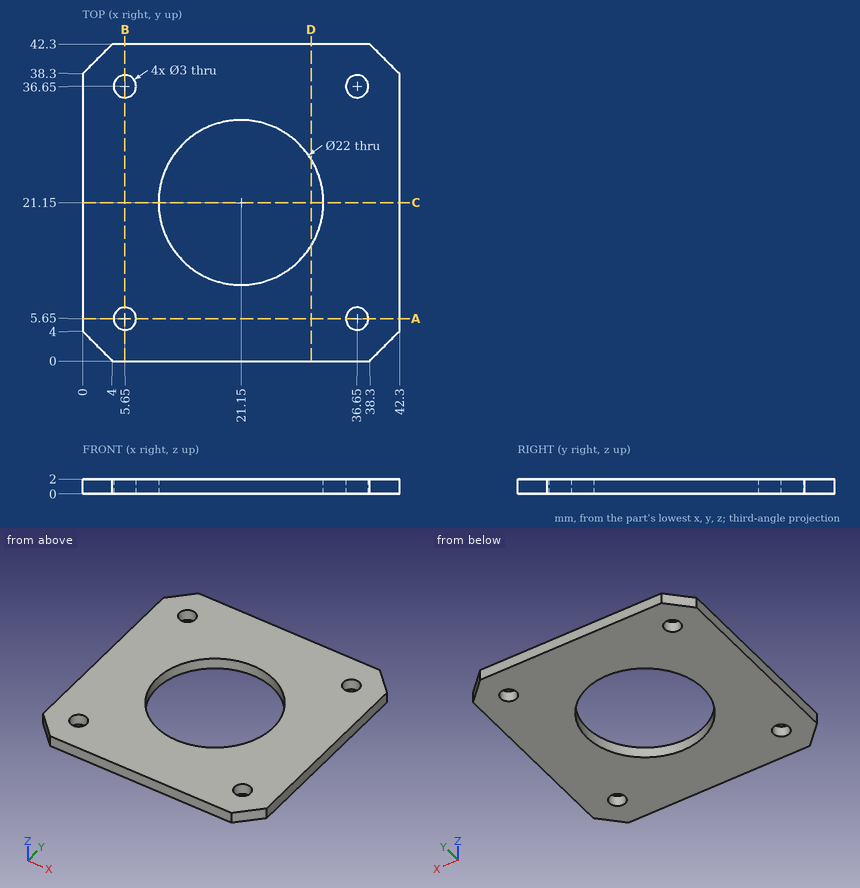
Design review of the part shown in the three views and the two pictorial views. Dimensions are in mm from the part's minimum x, y and z. Coordinates: 2 decimals unless noted, no trailing zeros. Order: outer loops, then holes, each group sorted by start corner. A loop starts at its lowest first (then second) coordinate and runs counter-clockwise, first axis right, second up. Notation, with made-up numbers: (-34.75, 57) - (5.25, 57) arc R5 ccw to (5.25, 61) - close; hole circle Ø9 at (-35, 69). An arc over 180 degrees is marked (long way). Answer as CSV lines item,"result". Start each with the question number.
1) Add section D-D (x = 30.5). State the section outline as (y, z) points.
2) Add section A-A (y = 5.65). State the section outline as (x, z) points, then the cut area to 3 significant figures.
3) Add section C-C (y = 21.15). State the section outline as (x, z) points, then the cut area to 3 significant figures.
4) Insertion check: P1, Ø3.5, axis at x = 36.65, y = 36.65, coming from the -Z side; P2, Ø1.8, axis at x = 5.65, y = 5.65, coming from the +Z side. Each pin has a flat end and moves straight along its axis. Give the tip position at first contact, or say it passes through.
5) To check wall thickness, follow line 1 along Y through (x, z) = (36.65, 1.1); line 2 along X through (y, z) = (21, 1); line 3 along Y through (x, z) = (21.5, 0.95). State the ranges of each line that lie inside material, in increasing order. Write a range as [from, to].
Result:
1,outline,"(0, 0) - (15.36, 0) - (15.36, 2) - (0, 2) - close; (26.94, 0) - (42.3, 0) - (42.3, 2) - (26.94, 2) - close"
2,outline,"(0, 0) - (4.15, 0) - (4.15, 2) - (0, 2) - close; (7.15, 0) - (35.15, 0) - (35.15, 2) - (7.15, 2) - close; (38.15, 0) - (42.3, 0) - (42.3, 2) - (38.15, 2) - close"
2,area,"72.6 mm^2"
3,outline,"(0, 0) - (10.15, 0) - (10.15, 2) - (0, 2) - close; (32.15, 0) - (42.3, 0) - (42.3, 2) - (32.15, 2) - close"
3,area,"40.6 mm^2"
4,P1,"z = 0"
4,P2,"through"
5,line 1,"[0, 4.15], [7.15, 35.15], [38.15, 42.3]"
5,line 2,"[0, 10.15], [32.15, 42.3]"
5,line 3,"[0, 10.16], [32.14, 42.3]"
